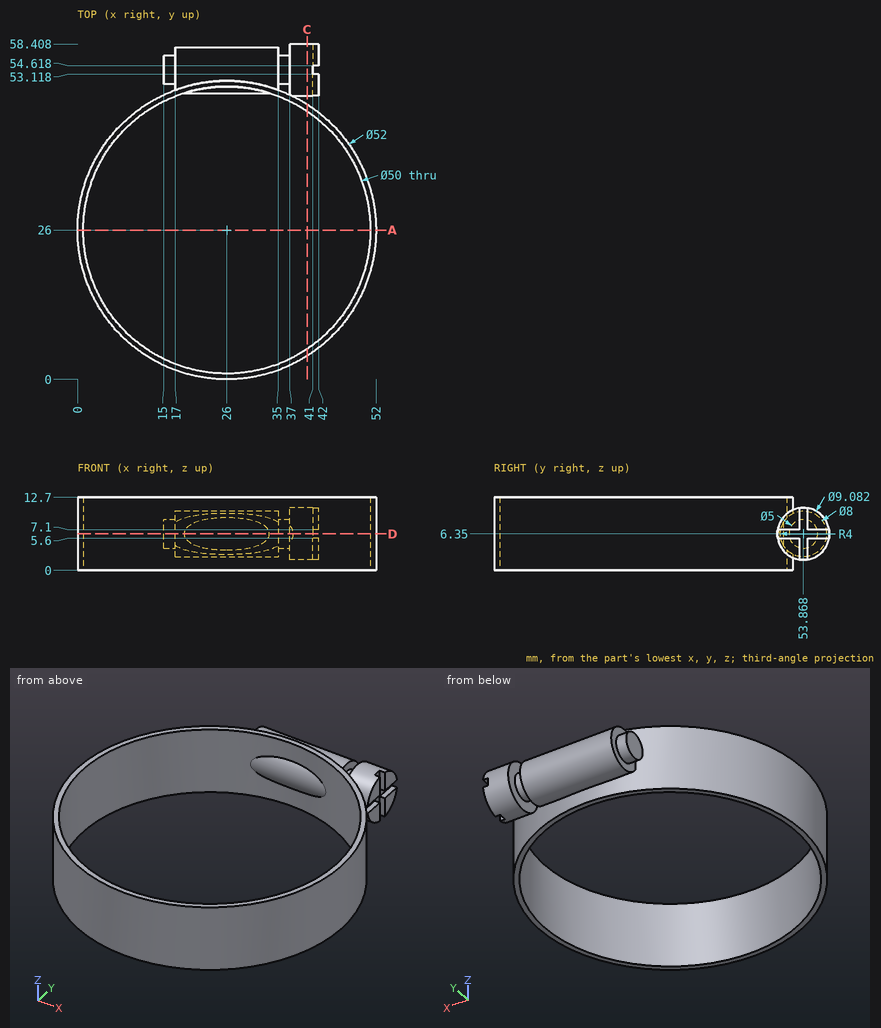
Geometry: see drawing. Coordinates: mm, zero at the bounding-box minimum. Round coordinates to 2 decimals unless told otherwise and drop trailing zeros. Loops run counter-clockwise (first coordinate to the right, second up) from the corner with the lowest first, then second, coordinate; pieces in that order, holes last. Notation, with made-up numbers: (-14.5, -8.5) - (15.5, -8.5) arc R22 ccw to (15.5, 3.5) - close; hole circle Ø11 at (38, 0). An arc over 180 degrees is marked (long way). One line per item, written item: value. Start each with the question number.
(1) Section C-C, the plane x = 40. Return loops of the section in (y, z).
(2) Section A-A, the plane y = 26. Return loops of the section in (x, z), plus the area to 3 significant figures.
(3) Contact query for flat-ended pins moving along their axis: P1, Ø1.1, axis at x = 41.5, z = 4, coming from the +Y side; P2, Ø1.1, axis at y = 51, z = 4.5, coming from the +X side; P3, Ø1.1, axis at x = 41.5, y = 50.5, coming from the -Z side. Output: stop coordinate, or through.
(4) Ray query, line 1 (Y direction, x = 26, z = 6); line 2 (Y direction, x = 40, z = 4) (1 decimal); line 3 (X direction, y = 8, z = 11.75). Return the intervals inside material, ascending. Write a range as [from, to].
(5) Section D-D, the plane z = 6.35. Return loops of the section in (x, y), plus the area to 3 significant figures.
Results below:
1. outline: (4.09, 0) - (5.29, 0) - (5.29, 12.7) - (4.09, 12.7) - close; (46.71, 0) - (47.91, 0) - (47.91, 12.7) - (46.71, 12.7) - close; circle Ø9.08 at (53.87, 6.35)
2. outline: (0, 0) - (1, 0) - (1, 12.7) - (0, 12.7) - close; (51, 0) - (52, 0) - (52, 12.7) - (51, 12.7) - close
2. area: 25.4 mm^2
3. P1: y = 58.04
3. P2: x = 42
3. P3: z = 2.79
4. line 1: [0, 1], [49.88, 57.85]
4. line 2: [4.1, 5.3], [46.7, 47.9], [50, 57.8]
4. line 3: [7.24, 8.65], [43.35, 44.76]
5. outline: (15, 51.37) - (17, 51.37) - (17, 50.39) arc R26 ccw (long way) to (37.48, 49.33) - (41, 49.33) - (41, 58.41) - (37, 58.41) - (37, 56.37) - (35, 56.37) - (35, 57.87) - (17, 57.87) - (17, 56.37) - (15, 56.37) - close; hole (18.56, 49.87) arc R25 ccw (long way) to (33.44, 49.87) - close; hole (35, 50.39) arc R26 cw to (37, 49.56) - (37, 51.37) - (35, 51.37) - close
5. area: 343 mm^2
